Model file for the job. Use its own axes, mm. Face numbers are marked on the shaded views. A direction names the side the tool comes from. Coordinates: 2 decimals unless noted, no trailing zeros. Write each loop counter-clockwise with the first axis right and the second up, starting at its lowest first coordinate (ties: lowest second). Pieces come first, ordered by that corner, then holes. Notation, with made-up numbers: (-25.5, 8) - (5.5, 8) arc R34 ccw to (5.5, 38) - close; hole circle Ø10 at (46, 78.5). An arc over 180 degrees is marked (long way). Put each result on its own line as item: value. Start each with the question number.
1. Pull direction X, two halves, no side cores. Call the marked faces 1, 2 and 3: released by +X, released by -X, zero draft, split by the parting line, or undercut.
2. Saw through at D-D, the plane x = -16.5. Write the cut outline in (y, z).
3. Drop flat-ended pins along their axis: P1, Ø1.2, axis at x = -12, z = 0.5, coming from the -Y side; P2, Ø2, axis at x = -11, y = -6.5, coming from the -Z side. Give the stop position or say it passes through.
4. Which spindle directions (+Z, -Z, +X, -X, +Y, -Y) get a long thin tool onto all of the face, cutting with end or side? Do the marked faces 4, 5 and 6. Say none if no direction does.
5. Saw through at A-A, the plane y = -6. Give the number of separate pieces and of enclosed holes in the cut face, plus the area to 3 significant figures.
6. Drill centre lines: L1, parallel to Z at x = 16.5, y = -5.9; L2, parallel to Z at x = 11, y = -7.05; L3, parallel to Z at x = 0, y = -6.25. Where is each one in solid material? Low to high. Write a range as from..to.
7. Saw through at B-B, the plane x = 0. Write the cut outline in (y, z), plus the area to 3 significant figures.
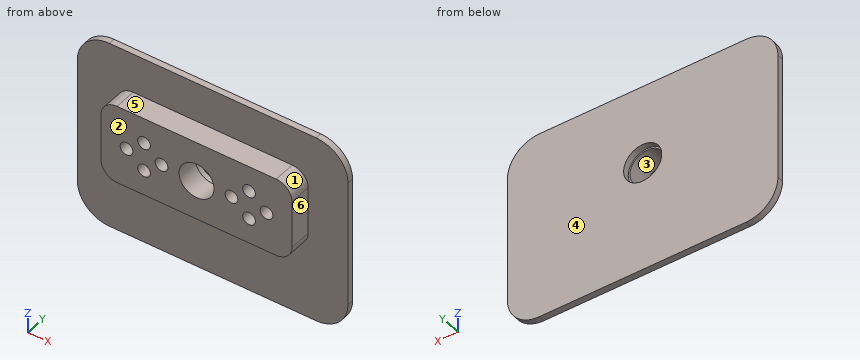
```python
from build123d import *

# Parameters (mm, degrees)
F0_W     = 85
F0_H     = 60
F0_R     = 6
F1_DEPTH = 2
F2_W     = 60
F2_H     = 25
F2_R     = 5.5
F3_DEPTH = 7
F4_R     = 5
F5_R     = 10
F6_R     = 2
F7_DEPTH = 4


with BuildPart() as f1:
    # F0 (on Front) → F1 (new body)
    with BuildSketch(Plane.XZ):
        with Locations((0, -5)):
            Rectangle(F0_W, F0_H)
        Circle(F0_R, mode=Mode.SUBTRACT)
    extrude(amount=F1_DEPTH)

    # F2 (on face) → F3 (join)
    with BuildSketch(Plane.XZ.offset(2)):
        Rectangle(F2_W, F2_H)
        Circle(F2_R, mode=Mode.SUBTRACT)
    extrude(amount=F3_DEPTH)

    # F4
    f4_edges = [f1.edges().sort_by_distance(p)[0] for p in [
        (30, -5.5, 12.5),
        (30, -5.5, -12.5),
        (-30, -5.5, -12.5),
        (-30, -5.5, 12.5),
    ]]
    fillet(f4_edges, radius=F4_R)

    # F5
    f5_edges = [f1.edges().sort_by_distance(p)[0] for p in [
        (42.5, -1, 25),
        (42.5, -1, -35),
        (-42.5, -1, -35),
        (-42.5, -1, 25),
    ]]
    fillet(f5_edges, radius=F5_R)

    # F6 (on face) → F7 (cut)
    with BuildSketch(Plane.XZ.offset(9)):
        with Locations((-11, 0)):
            Circle(F6_R)
        with Locations((-22, 0)):
            Circle(F6_R)
        with Locations((11, 0)):
            Circle(F6_R)
        with Locations((22, 0)):
            Circle(F6_R)
        with Locations((-16.5, -4.5)):
            Circle(F6_R)
        with Locations((16.5, -4.5)):
            Circle(F6_R)
        with Locations((16.5, 4.5)):
            Circle(F6_R)
        with Locations((-16.5, 4.5)):
            Circle(F6_R)
    extrude(amount=-F7_DEPTH, mode=Mode.SUBTRACT)


solid = f1.part
```
Final values:
1. face 1: released by +X
1. face 2: zero draft
1. face 3: undercut
2. outline: (-9, -12.5) - (-2, -12.5) - (-2, -35) - (0, -35) - (0, 25) - (-2, 25) - (-2, 12.5) - (-9, 12.5) - (-9, 6.5) - (-5, 6.5) - (-5, 2.5) - (-9, 2.5) - (-9, -2.5) - (-5, -2.5) - (-5, -6.5) - (-9, -6.5) - close
3. P1: stops at y = -5
3. P2: stops at z = -12.5
4. face 4: +Z, -Z, +X, -X, +Y
4. face 5: +Z, +X, -X, -Y
4. face 6: +Z, -Z, +X, -Y
5. separate pieces: 1
5. enclosed holes: 9
5. area: 1,280 mm²
6. L1: z = -12.5..-6.5, -2.5..2.5, 6.5..12.5
6. L2: z = -12.5..-2, 2..12.5
6. L3: z = -12.5..-5.5, 5.5..12.5
7. outline: (-9, -12.5) - (-2, -12.5) - (-2, -35) - (0, -35) - (0, -6) - (-2, -6) - (-2, -5.5) - (-9, -5.5) - close; (-9, 5.5) - (-2, 5.5) - (-2, 6) - (0, 6) - (0, 25) - (-2, 25) - (-2, 12.5) - (-9, 12.5) - close
7. area: 194 mm²
